```python
from build123d import *

# Parameters (mm, degrees)
F0_W     = 5.842
F0_H     = 12.7
F0_R     = 3.175
F1_DEPTH = 3.175
F4_DEPTH = 1.27
F3_R     = 1.524
F5_DEPTH = 56.134
F6_DEPTH = 6.35


with BuildPart() as f1:
    # F0 (on Front) → F1 (new body, symmetric)
    with BuildSketch(Plane.XZ):
        with BuildLine():
            Line((-0.9398, 0), (0, 0))
            Line((0, 0), (0, 12.7))
            Line((0, 12.7), (5.842, 12.7))
            Line((5.842, 12.7), (5.842, 15.24))
            Line((5.842, 15.24), (-0.508, 15.24))
            Line((-0.508, 15.24), (-10.8806298187, 3.8475430269))
            ThreePointArc((-10.8806298187, 3.8475430269), (-4.5919612295, 5.3297205562), (-0.9398, 0))
        make_face()
        with Locations((2.921, 6.35)):
            Rectangle(F0_W, F0_H)
        with BuildLine():
            ThreePointArc((-8.1826630726, -5.5069827884), (-3.1957909266, -4.5493385486), (-0.9398, 0))
            ThreePointArc((-0.9398, 0), (-4.5919612295, 5.3297205562), (-10.8806298187, 3.8475430269))
            ThreePointArc((-10.8806298187, 3.8475430269), (-12.1459778134, -1.5837270034), (-8.1826630726, -5.5069827884))
        make_face()
        with Locations((-6.6548, 0)):
            Circle(F0_R, mode=Mode.SUBTRACT)
        with BuildLine():
            Line((5.842, 0), (0, 0))
            Line((0, 0), (-0.9398, 0))
            ThreePointArc((-0.9398, 0), (-3.1957909266, -4.5493385486), (-8.1826630726, -5.5069827884))
            Line((-8.1826630726, -5.5069827884), (5.842, -9.398))
            Line((5.842, -9.398), (5.842, 0))
        make_face()
    extrude(amount=F1_DEPTH, both=True)

    # F0 (on Front) → F2 (revolve)
    with BuildSketch(Plane.XZ):
        Polygon((5.842, 12.7), (5.842, 0), (66.294, 0), (66.294, 12.7), (56.134, 12.7), (56.134, 10.16), (10.16, 10.16), (10.16, 12.7), align=None)
        with Locations((2.921, 6.35)):
            Rectangle(F0_W, F0_H)
    revolve(axis=Axis((33.147, 0, 0), (-1, 0, 0)))

    # F3 (on face) → F4 (join)
    with BuildSketch(Plane.YZ.offset(66.294)):
        with BuildLine():
            ThreePointArc((-5.08, 11.6397422652), (0, 12.7), (5.08, 11.6397422652))
            Line((5.08, 11.6397422652), (5.08, 15.24))
            Line((5.08, 15.24), (-5.08, 15.24))
            Line((-5.08, 15.24), (-5.08, 11.6397422652))
        make_face()
    extrude(amount=-F4_DEPTH)

    # F3 (on face) → F5 (cut, through all)
    with BuildSketch(Plane.YZ.offset(66.294)):
        Circle(F3_R)
    extrude(amount=-F5_DEPTH, mode=Mode.SUBTRACT)

    # F3 (on face) → F6 (join)
    with BuildSketch(Plane.YZ.offset(66.294)):
        with BuildLine():
            ThreePointArc((-5.08, 0), (0, -5.08), (5.08, 0))
            ThreePointArc((5.08, 0), (0, 5.08), (-5.08, 0))
        make_face()
        Circle(F3_R, mode=Mode.SUBTRACT)
        with BuildLine():
            ThreePointArc((-5.08, 0), (0, 5.08), (5.08, 0))
            Line((5.08, 0), (5.08, 11.6397422652))
            ThreePointArc((5.08, 11.6397422652), (0, 12.7), (-5.08, 11.6397422652))
            Line((-5.08, 11.6397422652), (-5.08, 0))
        make_face()
        with BuildLine():
            ThreePointArc((-5.08, 11.6397422652), (0, 12.7), (5.08, 11.6397422652))
            Line((5.08, 11.6397422652), (5.08, 15.24))
            Line((5.08, 15.24), (-5.08, 15.24))
            Line((-5.08, 15.24), (-5.08, 11.6397422652))
        make_face()
    extrude(amount=F6_DEPTH)


solid = f1.part
```
Input: part model. Units: mm. Frame: model coordinates. A direction names the side the tool comes from. Round coordinates to 2 decimals unless told otherwise and drop trailing zeros. Loops run counter-clockwise (first coordinate to the right, second up) from the corner with the lowest first, then second, coordinate; pieces in that order, holes last. Notation, with made-up numbers: (-16.5, -31) - (38.5, -31) arc R17 cw to (38.5, -11) - close; hole circle Ø7 at (-17, 61.5). An arc over 180 degrees is marked (long way). One line per item, written item: value. Start each with the question number.
(1) Contact query for flat-ended pins moving along their axis: P1, Ø5, axis at y = -10, z = 4.5, coming from the +X side; P2, Ø5.5, axis at x = -3, z = 2.5, coming from the +Y side (3 decimals); P3, Ø3, axis at x = 29.5, z = 4, coming from the +Y side. Output: stop coordinate, or through.
(2) Section C-C, the plane y = 4.25. Return loops of the section in (x, z).
(3) Section B-B, the plane x = 57. Return loops of the section in (y, z), plus the area to 3 significant figures.
(4) Access query for faces 1 (the flat face through (66.294, 0, -6)), 2 (the flat face through (69, 0, 15.24)), 3 (the flat face through (-4.149, -0.044, -6.626)), 4 (the flat face through (10.16, 0, 0)), 5 (the cylindrical face through (32.825, 10.074, -1.323)). Directions: +Z, -Z, +X, -X, +Y, -Y. A direction counts if a zero-diameter tool reaches every point of the face in a straight line with its end or side. Return the directions, or none.
(5) Section A-A, the plane y = 0. Return loops of the section in (x, z) (3 decimals), plus the area to 3 significant figures.
(6) Ray query, line 1 (X direction, y = 11.5, z = -3.75); line 2 (X direction, y = 1, z = -0.5); line 3 (X direction, y = -6.25, z = 3.75). Return the intervals inside material, ascending. Write a range as [from, to].
(7) Section D-D, the plane x = -1.5. Return loops of the section in (y, z) (3 decimals), plus the area to 3 significant figures.
(8) Draft query along X for faces 6 (the flat face through (-3, -3.175, 4)), 7 (the flat face through (72.644, 0, 5)), 8 (the cylindrical face through (-3.626, 0.044, 0.954)). Return one class per face: +X half, -X half, draft (parallel to the pull), parting line (faces both ways), or undercut.
Results below:
1. P1: x = 66.29
1. P2: y = 3.175
1. P3: y = 9.85
2. outline: (0, -11.97) - (10.16, -11.97) - (10.16, -9.23) - (56.13, -9.23) - (56.13, -11.97) - (66.29, -11.97) - (66.29, -2.78) - (72.64, -2.78) - (72.64, 15.24) - (65.02, 15.24) - (65.02, 11.97) - (56.13, 11.97) - (56.13, 9.23) - (10.16, 9.23) - (10.16, 11.97) - (0, 11.97) - close
3. outline: circle Ø25.4 at (0, 0); hole circle Ø3.05 at (0, 0)
3. area: 499 mm^2
4. face 1: -Z, +X
4. face 2: +Z, +X, -X, +Y, -Y
4. face 3: -Z, -X, +Y, -Y
4. face 4: +X
4. face 5: none
5. outline: (-10.881, 3.848) arc R5.715 ccw to (-8.183, -5.507) - (0, -7.777) - (0, -12.7) - (10.16, -12.7) - (10.16, -10.16) - (56.134, -10.16) - (56.134, -12.7) - (66.294, -12.7) - (66.294, -5.08) - (72.644, -5.08) - (72.644, -1.524) - (10.16, -1.524) - (10.16, 1.524) - (72.644, 1.524) - (72.644, 15.24) - (65.024, 15.24) - (65.024, 12.7) - (56.134, 12.7) - (56.134, 10.16) - (10.16, 10.16) - (10.16, 12.7) - (5.842, 12.7) - (5.842, 15.24) - (-0.508, 15.24) - close; hole circle Ø6.35 at (-6.655, 0)
5. area: 1,560 mm^2
6. line 1: [0, 10.16], [56.13, 66.29]
6. line 2: [-12.35, -9.79], [-3.52, 10.16]
6. line 3: [0, 66.29]
7. outline: (-3.175, -7.361) - (3.175, -7.361) - (3.175, 14.15) - (-3.175, 14.15) - close
7. area: 137 mm^2
8. face 6: draft
8. face 7: +X half
8. face 8: undercut
